Source: CAD feature listing. Evaluate the final solid. Frame: model axes, mm. Face numbers are marked on the shaded views. A direction names the side the tool comes from. Give positions to 0.01 mm unless a question says otherwise; leave off trailing zeros. Order: outer loops, then holes, each group sorted by start corner. A loop starts at its lowest first (then second) coordinate and runs counter-clockwise, first axis right, second up. Notation, with made-up numbers: (-5.75, 62) - (-1.75, 62) arc R21 ccw to (-1.75, 101) - close; hole circle Ø8 at (23, -30). An arc over 180 degrees is marked (long way). Use CSV: the item, a comma, the result in double quotes.
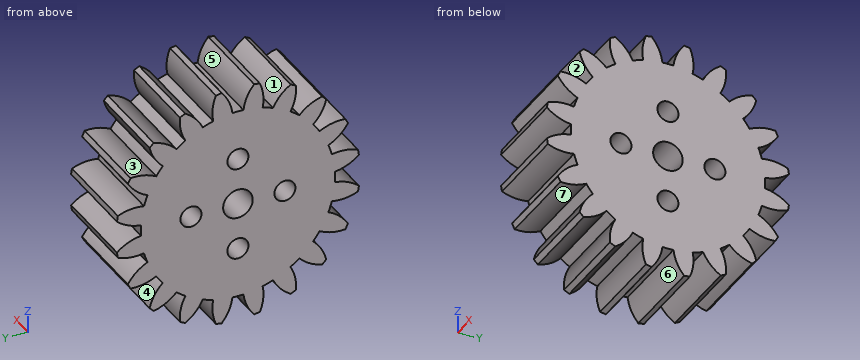
```python
from build123d import *

# Parameters (mm, degrees)
BASPROSKE_W        = 12
BASPROSKE_H        = 16.5
TOOTHCUT_DEPTH     = 27.239283527
TEETHCUTS_COUNT    = 20
TEETHCUTS_ANGLE    = 342
BORSKE_R           = 2
BORE_DEPTH         = 50.0000508
SKETCH1_R          = 1.4224
CUT_EXTRUDE1_DEPTH = 27.055895681


with BuildPart() as part:
    # BasProSke → Base-Revolve (revolve)
    with BuildSketch(Plane(origin=(0, 0, 0), x_dir=(1, 0, 0), z_dir=(0, 1, 0)), mode=Mode.PRIVATE) as base_revolve_sk:
        with Locations((6, 8.25)):
            Rectangle(BASPROSKE_W, BASPROSKE_H)
    revolve(base_revolve_sk.sketch.rotate(Axis((-10, 0, 0), (1, 0, 0)), 180), axis=Axis((-10, 0, 0), (1, 0, 0)))

    # TooCutSke → ToothCut (cut, through all)
    with BuildSketch(Plane(origin=(0, 0, 0), x_dir=(0, 0, -1), z_dir=(1, 0, 0))):
        with BuildLine():
            ThreePointArc((0.74381438, 13.102904875), (0, 13.124), (-0.74381438, 13.102904875))
            ThreePointArc((-0.74381438, 13.102904875), (-1.226473103, 14.852072512), (-2.209965745, 16.376962373))
            ThreePointArc((-2.209965745, 16.376962373), (0, 16.5254), (2.209965745, 16.376962373))
            ThreePointArc((2.209965745, 16.376962373), (1.226473103, 14.852072512), (0.74381438, 13.102904875))
        make_face()
    toothcut = extrude(amount=TOOTHCUT_DEPTH, mode=Mode.SUBTRACT)

    # TeethCuts: ToothCut ×20 about axis
    teethcuts_axis = Axis((-10, 0, 0), (1, 0, 0))
    for i in range(1, TEETHCUTS_COUNT):
        add(toothcut.rotate(teethcuts_axis, i * TEETHCUTS_ANGLE / (TEETHCUTS_COUNT - 1)), mode=Mode.SUBTRACT)

    # BorSke → Bore (cut, symmetric)
    with BuildSketch(Plane(origin=(0, 0, 0), x_dir=(0, 0, -1), z_dir=(1, 0, 0))):
        with Locations(Location((0, 0, 0), (0, 0, 180))):
            Circle(BORSKE_R)
    extrude(amount=BORE_DEPTH, both=True, mode=Mode.SUBTRACT)

    # Sketch1 → Cut-Extrude1 (cut, through all)
    with BuildSketch(Plane(origin=(0, 0, 0), x_dir=(0, 0, -1), z_dir=(1, 0, 0))):
        with Locations((0, 6.35)):
            Circle(SKETCH1_R)
        with Locations((6.35, 0)):
            Circle(SKETCH1_R)
        with Locations((0, -6.35)):
            Circle(SKETCH1_R)
        with Locations((-6.35, 0)):
            Circle(SKETCH1_R)
    extrude(amount=CUT_EXTRUDE1_DEPTH, mode=Mode.SUBTRACT)


solid = part.part
```
Item 1: First-contact query: pin 1 (2 mm diameter, centred on x = 10.5, z = 4.5, fed in from -Y); pin 2 (2 mm diameter, centred on x = 7, y = -8, fed in from -Z); pin 3 (1 mm diameter, centred on x = 2, z = 7.5, fed in from -Y). Flat tips, straight axial feed; report the tip coordinate or a pass-through.
Filled in:
pin 1,"stops at y = -13.44"
pin 2,"stops at z = -14.88"
pin 3,"stops at y = -14.88"
Item 2: Mould query, pull axis Z, two halves, no side actions, for the marked faces 5, 6 and 7. Classes: released by +Z, released by -Z, zero draft, split by the parting line, or undercut.
Filled in:
face 5,"released by +Z"
face 6,"released by -Z"
face 7,"undercut"
Item 3: Material intervals for line 1 (Y direction, x = 9.75, z = 0); line 2 (Y direction, x = 10.5, z = 14); line 3 (Z direction, x = 11.75, y = 0.5), sorted ascending. Write a range as from..to.
Filled in:
line 1,"y = -13.12..-7.77, -4.93..-2, 2..4.93, 7.77..13.12"
line 2,"y = -7.87..-6, -3.46..-0.92, 0.92..3.46, 6..7.87"
line 3,"z = -13.11..-7.68, -5.02..-1.94, 1.94..5.02, 7.68..13.11"
Item 4: Set-up query: the marked faces 1, 2, 3 and 4. Return all of +Z, -Z, +X, -X, +Y, -Y with unobstructed straight access to the full face (end or side cutting, diameter ignored); none if empty.
Filled in:
face 1,"+Z, +X, -X"
face 2,"+X, -X, -Y"
face 3,"+X, -X"
face 4,"+X, -X, +Y"
Item 5: Section C-C on z = 6.35. Return the cut outline in (x, y), then the cut area to 3 significant figures.
Filled in:
outline,"(0, -14.32) - (12, -14.32) - (12, -1.42) - (0, -1.42) - close; (0, 1.42) - (12, 1.42) - (12, 14.32) - (0, 14.32) - close"
area,"310 mm2"
Item 6: Section A-A on y = 0. Return the cut outline in (x, z).
Filled in:
outline,"(0, -13.12) - (12, -13.12) - (12, -7.77) - (0, -7.77) - close; (0, -4.93) - (12, -4.93) - (12, -2) - (0, -2) - close; (0, 2) - (12, 2) - (12, 4.93) - (0, 4.93) - close; (0, 7.77) - (12, 7.77) - (12, 13.12) - (0, 13.12) - close"
